Answer from the drawing. Dimensions are ordinates in mm from the lowest x, y and z of the part. Coordinates: 2 decimals unless noted, no trailing zeros. Order: outer loops, then holes, each group sorted by start corner. A loop starts at its lowest first (then second) coordinate and runs counter-clockwise, first axis right, second up. Notation, with made-up numbers: (-29, 40.5) - (-22, 40.5) arc R17 cw to (-22, 62.5) - close; hole circle Ø7 at (35, 49.5). An arc over 180 degrees is marked (long way). Answer as a JSON object with one key per item and string values. Group by question number.
1) Find the intervals of material crossed by line 1 along X through (y, z) = (3, 5.5); line 2 along X through (y, z) = (1.2, 6); line 3 along Z through (x, y) = (120, 4.65), in increasing order.
2) Each of these flat-tipped pins is pushed along its axis until it touches: P1, Ø1.5, axis at x = 69, y = 2.5, coming from the +Z side; P2, Ø2, axis at x = 85.5, y = 3.5, coming from the +Z side. Where does it stop, or does it pass through?
3) Section C-C (x = 108.5) is taken. Give the vertices of the cut face in (y, z), plus the area to 3 significant figures.
4) Section B-B (x = 77.5) is taken. Give the vertices of the cut face in (y, z), plus the area to 3 significant figures.
5) Section A-A (z = 2.5) is taken. Give the vertices of the cut face in (x, y), plus the area to 3 significant figures.
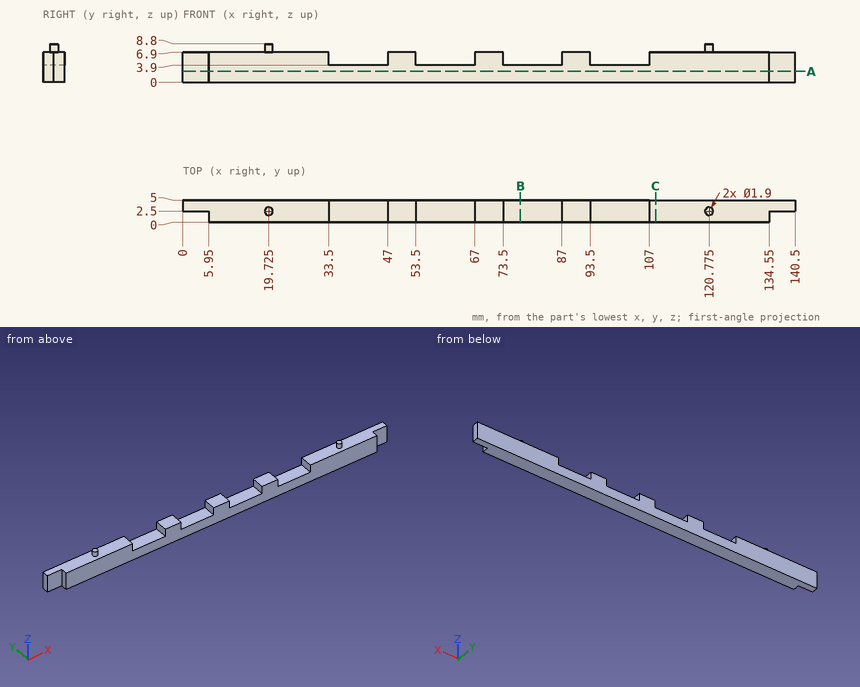
Report:
{
 "1": {"line 1": "x = 0 to 33.5, 47 to 53.5, 67 to 73.5, 87 to 93.5, 107 to 140.5", "line 2": "x = 5.95 to 33.5, 47 to 53.5, 67 to 73.5, 87 to 93.5, 107 to 134.55", "line 3": "z = 0 to 6.9"},
 "2": {"P1": "stops at z = 6.9", "P2": "stops at z = 3.9"},
 "3": {"outline": "(0, 0) - (5, 0) - (5, 6.9) - (0, 6.9) - close", "area": "34.5 mm²"},
 "4": {"outline": "(0, 0) - (5, 0) - (5, 3.9) - (0, 3.9) - close", "area": "19.5 mm²"},
 "5": {"outline": "(0, 2.5) - (5.95, 2.5) - (5.95, 0) - (134.55, 0) - (134.55, 2.5) - (140.5, 2.5) - (140.5, 5) - (0, 5) - close", "area": "673 mm²"}
}
